The model under review builds one solid part; all positions refer to its coordinate system, in mm. Face numbers are marked on the shaded views. A direction names the side the tool comes from. Coordinates: 2 decimals unless noted, no trailing zeros. Write each loop counter-clockwise with the first axis right and the second up, starting at its lowest first coordinate (ties: lowest second). Pieces come first, ordered by that corner, then holes.
1) Machinability: for the marked faces 1 and 2, which of the approach directions +Z, -Z, +X, -X, +Y, -Y give a long, thin tool a straight path to every point of the face, cutting with its end or side? Answer none if there is none.
2) Add section D-D, the plane x = 5.25. State the section outline as (y, z) points.
3) For P1, Ø1, axis at y = 6.5, z = -6.5, coming from the -X side; P2, Ø2, axis at x = 5.66, z = -5.66, coming from the -Y side; P3, Ø1.3, axis at x = 6.5, z = -5, coming from the +Y side; P4, Ø4, axis at x = -4, y = 9, coming from the -Z side, all flat-tipped, find the tip position at first contact; note any pin that passes through.
4) Mouldability with a two-part tool opening along Z and no side actions: class the marked faces 3, 4 and 5 as released by +Z, released by -Z, zero draft, split by the parting line, or undercut.
5) For line 1 (Y direction, x = -5.5, z = -9.25); line 2 (Z direction, x = -4.5, y = 2.75); line 3 (X direction, y = 4.5, z = -5.25), list the stretches that pass through material, from the lowest coordinate up.
6) Add section C-C, the plane z = -7.5. State the section outline as (x, y) points, then the cut area to 3 significant figures.
7) Add section A-A, the plane y = 5. Give the number of separate pieces and of enclosed holes in the cut face, then the cut area to 3 significant figures.
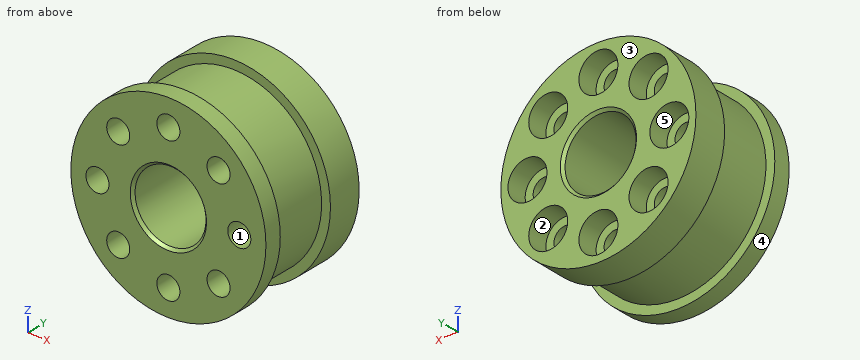
from build123d import *

# Parameters (mm, degrees)
SKETCH1_R                                           = 11
BOSS_EXTRUDE1_DEPTH                                 = 13
CBORE_FOR_M2_HEX_SOCKET_HEAD_CAP_SCREW1_D           = 2.6
CBORE_FOR_M2_HEX_SOCKET_HEAD_CAP_SCREW1_CBORE_D     = 4.4
CBORE_FOR_M2_HEX_SOCKET_HEAD_CAP_SCREW1_CBORE_DEPTH = 2.4
CUT_EXTRUDE1_START                                  = -2
SKETCH8_R                                           = 11
SKETCH8_R_2                                         = 10
CUT_EXTRUDE1_DEPTH                                  = 7


with BuildPart() as part:
    # Sketch1 → Boss-Extrude1 (new body)
    with BuildSketch(Plane(origin=(0, 0, 0), x_dir=(1, 0, 0), z_dir=(0, 1, 0))):
        with Locations(Location((0, 0, 0), (0, 0, 90))):
            Circle(SKETCH1_R)
    extrude(amount=BOSS_EXTRUDE1_DEPTH)

    # CBORE for M2 Hex Socket Head Cap Screw1 (through all)
    with Locations(Plane(origin=(0, 13, 0), x_dir=(1, 0, 0), z_dir=(0, 1, 0))):
        with Locations((-5.656854249, 5.656854249), (0, 8), (5.656854249, 5.656854249), (8, 0), (5.656854249, -5.656854249), (0, -8), (-5.656854249, -5.656854249), (-8, 0)):
            CounterBoreHole(CBORE_FOR_M2_HEX_SOCKET_HEAD_CAP_SCREW1_D / 2, CBORE_FOR_M2_HEX_SOCKET_HEAD_CAP_SCREW1_CBORE_D / 2, CBORE_FOR_M2_HEX_SOCKET_HEAD_CAP_SCREW1_CBORE_DEPTH)

    # Sketch8 → Cut-Extrude1 (cut)
    with BuildSketch(Plane.XZ.offset(CUT_EXTRUDE1_START)):
        with Locations(Location((0, 0, 0), (0, 0, 270))):
            Circle(SKETCH8_R)
        with Locations(Location((0, 0, 0), (0, 0, 270))):
            Circle(SKETCH8_R_2, mode=Mode.SUBTRACT)
    extrude(amount=-CUT_EXTRUDE1_DEPTH, mode=Mode.SUBTRACT)

    # Sketch12 → Ø8.0mm Dowel Hole1 (revolve, cut)
    with BuildSketch(Plane(origin=(0, 0, 0), x_dir=(0, 0, -1), z_dir=(1, 0, 0))):
        Polygon((0, 0), (0, 13), (4.3, 13), (4, 12.7), (4, 0.3), (4.3, 0), align=None)
    revolve(axis=Axis((0, -6.35, 0), (0, 1, 0)), mode=Mode.SUBTRACT)


solid = part.part
Geometry results:
1. face 1: +Y, -Y
1. face 2: +Y
2. outline: (0, -9.67) - (2, -9.67) - (2, -8.51) - (9, -8.51) - (9, -9.67) - (13, -9.67) - (13, -7.82) - (10.6, -7.82) - (10.6, -6.89) - (0, -6.89) - close; (0, -4.42) - (10.6, -4.42) - (10.6, -3.49) - (13, -3.49) - (13, 3.49) - (10.6, 3.49) - (10.6, 4.42) - (0, 4.42) - close; (0, 6.89) - (10.6, 6.89) - (10.6, 7.82) - (13, 7.82) - (13, 9.67) - (9, 9.67) - (9, 8.51) - (2, 8.51) - (2, 9.67) - (0, 9.67) - close
3. P1: stops at x = -8
3. P2: passes through
3. P3: stops at y = 10.6
3. P4: stops at z = -10.82
4. face 3: zero draft
4. face 4: split by the parting line
4. face 5: undercut
5. line 1: y = 0 to 2, 9 to 13
5. line 2: z = -8.93 to -6.25, -5.06 to 5.06, 6.25 to 8.93
5. line 3: x = -8.51 to -6.89, -4.42 to 4.42, 6.89 to 8.51
6. outline: (-8.05, 0) - (-1.2, 0) - (-1.2, 10.6) - (-2.14, 10.6) - (-2.14, 13) - (-4.46, 13) - (-4.46, 10.6) - (-6.86, 10.6) - (-6.86, 13) - (-8.05, 13) - (-8.05, 9) - (-6.61, 9) - (-6.61, 2) - (-8.05, 2) - close; (1.2, 0) - (8.05, 0) - (8.05, 2) - (6.61, 2) - (6.61, 9) - (8.05, 9) - (8.05, 13) - (6.86, 13) - (6.86, 10.6) - (4.46, 10.6) - (4.46, 13) - (2.14, 13) - (2.14, 10.6) - (1.2, 10.6) - close
6. area: 142 mm2
7. separate pieces: 1
7. enclosed holes: 9
7. area: 221 mm2
